Can you work these out from the model? Positions are in its coordinate system, mm. A direction names the side the tool comes from. Round coordinates to 2 decimals unless told otherwise and drop trailing zeros. Loops run counter-clockwise (first coordinate to the right, second up) from the corner with the lowest first, then second, coordinate; pieces in that order, holes last.
from build123d import *

# Parameters (mm, degrees)
F0_W     = 101.5
F0_H     = 10
F0_R     = 1.5
F0_W_2   = 66.5
F0_H_2   = 3
F0_R_2   = 2.5
F1_DEPTH = 3.5
F2_W     = 78.5
F2_H     = 10
F3_DEPTH = 0.5


with BuildPart() as f1:
    # F0 (on Front) → F1 (new body)
    with BuildSketch(Plane.XZ):
        Rectangle(F0_W, F0_H)
        with Locations((-34.75, -0.5)):
            Circle(F0_R, mode=Mode.SUBTRACT)
        with Locations((3, -0.5)):
            Rectangle(F0_W_2, F0_H_2, mode=Mode.SUBTRACT)
        with Locations((-45, 0)):
            Circle(F0_R_2, mode=Mode.SUBTRACT)
        with Locations((45, 0)):
            Circle(F0_R_2, mode=Mode.SUBTRACT)
    extrude(amount=F1_DEPTH)

    # F2 (on face) → F3 (cut)
    with BuildSketch(Plane.XZ.offset(3.5)):
        Rectangle(F2_W, F2_H)
    extrude(amount=-F3_DEPTH, mode=Mode.SUBTRACT)


solid = f1.part
(1) If I drill on line 1 (Z direction, x = -34.75, y = -2.15); line 2 (Z direction, x = -45, y = -2.5); line 3 (X direction, y = -2, z = -0.5), over which ranges is the centre line in solid material (lowest first)?
Worked answers:
line 1: z = -5 to -2, 1 to 5
line 2: z = -5 to -2.5, 2.5 to 5
line 3: x = -50.75 to -47.45, -42.55 to -36.25, -33.25 to -30.25, 36.25 to 42.55, 47.45 to 50.75
(2) Will this pin go through, and if not, where does the flat tip stop? P1, Ø3, axis at x = 5.5, z = 2.5, coming from the -Y side.
Worked answers:
P1: stops at y = -3
(3) If we section it at C-C, the plane x = 1: List the corners of the cut face in (y, z) for me, then the cut area to 3 significant figures.
Worked answers:
outline: (-3, -5) - (0, -5) - (0, -2) - (-3, -2) - close; (-3, 1) - (0, 1) - (0, 5) - (-3, 5) - close
area: 21.0 mm2
(4) If we section it at A-A, the plane x = -45: List the corners of the cut face in (y, z) for me.
Worked answers:
outline: (-3.5, -5) - (0, -5) - (0, -2.5) - (-3.5, -2.5) - close; (-3.5, 2.5) - (0, 2.5) - (0, 5) - (-3.5, 5) - close
(5) If we mould it in two halves opening along Z, with no side actions, what happens to faces 1 (the flat face through (-50.75, -2, 0)), 2 (the flat face through (-1, -2, 5)), 3 (the flat face through (-1, -2, -5)), 4 (the cylindrical face through (47.31, -1.73, -0.96))? For each: released by +Z, released by -Z, zero draft, split by the parting line, or undercut.
Worked answers:
face 1: zero draft
face 2: released by +Z
face 3: released by -Z
face 4: undercut
(6) For faces 5 (the flat face through (3, -1, 1)), 6 (the flat face through (-0.5, -3, 1.2)), 7 (the flat face through (-48, -3.5, 0)), which set-ups out of +Z, -Z, +X, -X, +Y, -Y let a thin tool reach every point of the face, with its end or its side?
Worked answers:
face 5: +Y, -Y
face 6: +Z, -Z, -Y
face 7: +Z, -Z, +X, -X, -Y
(7) If we section it at B-B, the plane y = -1.65: List the corners of the cut face in (x, z) for me, then the cut area to 3 significant figures.
Worked answers:
outline: (-50.75, -5) - (50.75, -5) - (50.75, 5) - (-50.75, 5) - close; hole circle Ø5 at (-45, 0); hole circle Ø3 at (-34.75, -0.5); hole (-30.25, -2) - (36.25, -2) - (36.25, 1) - (-30.25, 1) - close; hole circle Ø5 at (45, 0)
area: 769 mm2
